```python
from build123d import *

# Parameters (mm, degrees)
SKETCH1_R           = 1.5
SKETCH1_R_2         = 2
BOSS_EXTRUDE1_DEPTH = 3
FILLET1_R           = 4
FILLET2_R           = 10


with BuildPart() as part:
    # Sketch1 → Boss-Extrude1 (new body)
    with BuildSketch(Plane.XY):
        Polygon((-164.552800631, 70), (164.552800631, 70), (179, 70), (179, 50), (80, 50), (80, -50), (179, -50), (179, -70), (164.552800631, -70), (-164.552800631, -70), (-179, -70), (-179, -50), (-80, -50), (-80, 50), (-179, 50), (-179, 70), align=None)
        with Locations((-169, 60)):
            Circle(SKETCH1_R, mode=Mode.SUBTRACT)
        with Locations((-37.5, 37.5)):
            Circle(SKETCH1_R_2, mode=Mode.SUBTRACT)
        with Locations((37.5, 37.5)):
            Circle(SKETCH1_R_2, mode=Mode.SUBTRACT)
        with Locations((169, 60)):
            Circle(SKETCH1_R, mode=Mode.SUBTRACT)
        with Locations((169, -60)):
            Circle(SKETCH1_R, mode=Mode.SUBTRACT)
        with Locations((37.5, -37.5)):
            Circle(SKETCH1_R_2, mode=Mode.SUBTRACT)
        with Locations((-37.5, -37.5)):
            Circle(SKETCH1_R_2, mode=Mode.SUBTRACT)
        with Locations((-169, -60)):
            Circle(SKETCH1_R, mode=Mode.SUBTRACT)
    extrude(amount=BOSS_EXTRUDE1_DEPTH)

    # Fillet1
    fillet1_edges = [part.edges().sort_by_distance(p)[0] for p in [
        (179, 70, 1.5),
        (179, 50, 1.5),
        (179, -50, 1.5),
        (179, -70, 1.5),
        (-179, -70, 1.5),
        (-179, -50, 1.5),
        (-179, 50, 1.5),
        (-179, 70, 1.5),
    ]]
    fillet(fillet1_edges, radius=FILLET1_R)

    # Fillet2
    fillet2_edges = [part.edges().sort_by_distance(p)[0] for p in [
        (80, 50, 1.5),
        (80, -50, 1.5),
        (-80, -50, 1.5),
        (-80, 50, 1.5),
    ]]
    fillet(fillet2_edges, radius=FILLET2_R)


solid = part.part
```
Design review of the part built by this model. Coordinates are the model's own, in mm. A direction names the side the tool comes from. Give positions to 0.01 mm unless a question says otherwise; leave off trailing zeros. Order: outer loops, then holes, each group sorted by start corner. A loop starts at its lowest first (then second) coordinate and runs counter-clockwise, first axis right, second up. Notation, with made-up numbers: (77, 79.25) -> (125, 79.25) arc R23 ccw to (125, 109.25) -> close; hole circle Ø9 at (-39, 35.25). An arc over 180 degrees is marked (long way). Write item = value, one per line. Start each with the question number.
(1) To check wall thickness, follow line 1 along Y through (x, z) = (-169, 2.3); line 2 along Y through (x, z) = (37.5, 1.25); line 3 along Y through (x, z) = (116, 2.25). State the ranges of each line that lie inside material, in increasing order.
(2) We need section B-B on y = 13. Write out the cut boundary in (x, z), plus the area to 3 significant figures.
(3) For pin 1 (1.5 mm diameter, centred on y = 5, z = 1.5, fed in from -X), flat-tipped, find the tip position at first contact; note if it passes through.
(4) Mouldability with a two-part tool opening along Y and no side actions: class faces 1 (the face through (3, 1, 0)), 2 (the face through (-82.85, -46.99, 1.52)) as +Y half, -Y half, draft (parallel to the pull), parting line (faces both ways), or undercut.
(5) We need section A-A on z = 1.1. State how many separate pieces and enclosed holes the cut face has, plus the area to 3 significant figures.
(6) For faces 3 (the face through (83.01, 47.15, 1.52)), 4 (the face through (-83.01, 47.15, 1.52)), 5 (the face through (3, 1, 3)), list the 3-axis set-ups (+Z, -Z, +X, -X, +Y, -Y) from which the entire face can be reached by the end or side of a thin tool; tool diameter is ignored.
Numbers:
q1.line_1 = -70 to -61.5, -58.5 to -50, 50 to 58.5, 61.5 to 70
q1.line_2 = -70 to -39.5, -35.5 to 35.5, 39.5 to 70
q1.line_3 = -70 to -50, 50 to 70
q2.outline = (-80, 0) -> (80, 0) -> (80, 3) -> (-80, 3) -> close
q2.area = 480 mm^2
q3.pin_1 = -80
q4.face_1 = draft
q4.face_2 = undercut
q5.separate_pieces = 1
q5.enclosed_holes = 8
q5.area = 30,300 mm^2
q6.face_3 = +Z, -Z, +X
q6.face_4 = +Z, -Z, -X
q6.face_5 = +Z, +X, -X, +Y, -Y
